Check sheet for the modelled part. Datum: model origin and axes. Units: mm. A direction names the side the tool comes from. Round coordinates to 2 decimals unless told otherwise and drop trailing zeros. Write each loop counter-clockwise with the first axis right and the second up, starting at its lowest first coordinate (ties: lowest second). Pieces come first, ordered by that corner, then holes. Notation, with made-up numbers: (10, 47) -> (16, 47) arc R18 ccw to (16, 58) -> close; hole circle Ø5 at (50.25, 10). An arc over 180 degrees is marked (long way). Write item = value, one per line.
Autodesk Inventor part; units mm, degrees
ref_plane "YZ Plane" through (0, 0, 0) normal (1, 0, 0) x (0, 1, 0)
ref_plane "XZ Plane" through (0, 0, 0) normal (0, 1, 0) x (-1, 0, 0)
ref_plane "XY Plane" through (0, 0, 0) normal (0, 0, 1) x (1, 0, 0)
sketch "Sketch1" plane through (0, 0, 0) normal (0, 1, 0) x (-1, 0, 0)
  line L0 (73.3629, -5.9836) -> (60.8629, -5.9836)
  line L1 (60.8629, -5.9836) -> (60.8629, -18.4836)
  line L2 (60.8629, -18.4836) -> (73.3629, -18.4836)
  line L3 (73.3629, -18.4836) -> (73.3629, -5.9836)
  line L4 (107.9129, -0.7336) -> (40.3129, -0.7336)
  line L5 (40.3129, -23.7336) -> (107.9129, -23.7336)
  line L6 (77.3838, -12.2336) -> (49.3838, -12.2336) construction
  line L7 (67.1129, -2.25) -> (67.1129, -23.25) construction
  line L8 (81.1129, -9.7336) -> (107.9129, -9.7336)
  line L9 (107.9129, -14.7336) -> (81.1129, -14.7336)
  line L10 (48.1129, -23.7336) -> (48.1129, -0.7336)
  line L11 (46.3129, -0.7336) -> (46.3129, -23.7336)
  line L12 (52.6129, -10.7336) -> (40.3129, -10.7336)
  line L13 (52.6129, -13.7336) -> (40.3129, -13.7336)
  line L14 (101.1129, -15.2836) -> (99.6129, -15.2836)
  line L15 (99.6129, -15.2836) -> (99.6129, -9.1836)
  line L16 (99.6129, -9.1836) -> (101.1129, -9.1836)
  line L17 (79.1129, -0.7336) -> (79.1129, -23.7336)
  line L18 (81.1129, -23.7336) -> (81.1129, -0.7336)
  line L19 (55.1129, -0.7336) -> (55.1129, -23.7336)
  line L20 (79.1129, -13.7336) -> (73.3629, -13.7336)
  line L21 (73.3629, -10.7336) -> (79.1129, -10.7336)
  line L22 (60.8629, -13.7336) -> (55.1129, -13.7336)
  line L23 (55.1129, -10.7336) -> (60.8629, -10.7336)
  line L24 (73.3629, -18.4836) -> (77.5629, -18.4836)
  line L25 (77.5629, -18.4836) -> (77.5629, -15.2836)
  line L26 (77.5629, -15.2836) -> (73.3629, -15.2836)
  line L27 (73.3629, -15.2836) -> (60.8629, -15.2836)
  line L28 (56.2629, -15.2836) -> (56.2629, -18.4836)
  line L29 (56.2629, -18.4836) -> (59.4629, -18.4836)
  line L30 (59.4629, -15.2836) -> (56.2629, -15.2836)
  line L31 (59.4629, -5.9836) -> (56.2629, -5.9836)
  line L32 (56.2629, -5.9836) -> (56.2629, -9.1836)
  line L33 (56.2629, -9.1836) -> (59.4629, -9.1836)
  line L34 (60.8629, -9.1836) -> (73.3629, -9.1836)
  line L35 (77.5629, -9.1836) -> (77.5629, -5.9836)
  line L36 (73.3629, -5.9836) -> (77.5629, -5.9836)
  line L37 (77.5629, -9.1836) -> (73.3629, -9.1836)
  line L38 (59.4629, -18.4836) -> (59.4629, -15.2836)
  line L39 (59.4629, -9.1836) -> (59.4629, -5.9836)
  line L40 (60.8629, -18.4836) -> (59.4629, -18.4836)
  line L41 (60.8629, -15.2836) -> (59.4629, -15.2836)
  line L42 (60.8629, -9.1836) -> (59.4629, -9.1836)
  line L43 (60.8629, -5.9836) -> (59.4629, -5.9836)
  line L44 (40.3129, -23.7336) -> (40.3129, -0.7336)
  line L45 (107.9129, -23.7336) -> (107.9129, -0.7336)
  line L46 (53.1129, -14.7336) -> (52.6129, -14.7336)
  line L47 (52.6129, -14.7336) -> (52.6129, -9.7336)
  line L48 (52.6129, -9.7336) -> (53.1129, -9.7336)
  line L49 (53.1129, -23.7336) -> (53.1129, -14.7336)
  line L50 (53.1129, -9.7336) -> (53.1129, -0.7336)
  line L51 (101.1129, -16.2336) -> (98.1129, -16.2336)
  line L52 (98.1129, -16.2336) -> (98.1129, -18.2336)
  line L53 (98.1129, -18.2336) -> (101.1129, -18.2336)
  line L54 (102.9129, -16.2336) -> (105.9129, -16.2336)
  line L55 (105.9129, -16.2336) -> (105.9129, -18.2336)
  line L56 (105.9129, -18.2336) -> (102.9129, -18.2336)
  line L57 (101.1129, -8.2336) -> (98.1129, -8.2336)
  line L58 (98.1129, -8.2336) -> (98.1129, -6.2336)
  line L59 (98.1129, -6.2336) -> (101.1129, -6.2336)
  line L60 (102.9129, -8.2336) -> (105.9129, -8.2336)
  line L61 (105.9129, -8.2336) -> (105.9129, -6.2336)
  line L62 (105.9129, -6.2336) -> (102.9129, -6.2336)
  line L63 (106.4404, -17.2336) -> (97.7013, -17.2336) construction
  line L64 (106, -7.2336) -> (98, -7.2336) construction
  line L65 (102.9129, -23.7336) -> (102.9129, -18.2336)
  line L66 (101.1129, -18.2336) -> (101.1129, -23.7336)
  line L67 (102.9129, -16.2336) -> (102.9129, -8.2336)
  line L68 (102.9129, -6.2336) -> (102.9129, -0.7336)
  line L69 (101.1129, -0.7336) -> (101.1129, -6.2336)
  line L70 (101.1129, -8.2336) -> (101.1129, -16.2336)
  point P0 (102.9129, -9.7336)
  point P1 (101.1129, -9.7336)
  point P2 (102.9129, -14.7336)
  point P3 (101.1129, -14.7336)
  point P4 (48.1129, -10.7336)
  point P5 (46.3129, -10.7336)
  point P6 (48.1129, -13.7336)
  point P7 (46.3129, -13.7336)
  point P8 (67.1129, -12.2336)
  point P9 (99.6129, -9.7336)
  point P10 (99.6129, -14.7336)
  dimension "d0" = 12.5
  dimension "d1" = 12.5
  dimension "d12" = 5
  dimension "d18" = 1.8
  dimension "d39" = 1.5
  dimension "d43" = 2
  dimension "d52" = 12
  dimension "d57" = 12
  dimension "d62" = 3
  dimension "d63" = 3
  dimension "d71" = 7
  dimension "d76" = 4.2
  dimension "d77" = 3.2
  dimension "d78" = 3.2
  dimension "d79" = 1.4
  dimension "d80" = 3.2
  dimension "d91" = 6
  dimension "d92" = 3
  dimension "d95" = 23
  dimension "d98" = 5
  dimension "d99" = 0.5
  dimension "d100" = 2
  dimension "d101" = 2
  dimension "d102" = 3
  dimension "d103" = 10
  dimension "d104" = 1.8
  dimension "d105" = 20
  dimension "d107" = 6.1
  dimension "d108" = 5
  dimension "d109" = 67.6
extrude "Extrusion11" add sketch "Sketch1" against normal blind 3 contours L3 L34 L1 L0 | L1 L42 L39 L43 | L3 L2 L1 L27 | L1 L40 L38 L41
extrude "Extrusion10" add sketch "Sketch1" against normal blind 6 separate body contours L0 L43 L31 L32 L33 L42 L1 L23 L19 L4 L17 L21 L3 L37 L35 L36 | L3 L27 L1 L34 | L21 L17 L20 L3 | L1 L22 L19 L23 | L20 L17 L5 L19 L22 L1 L41 L30 L28 L29 L40 L2 L24 L25 L26 L3 | L17 L4 L18 L5 | L19 L5 L49 L46 L47 L48 L50 L4 | L4 L69 L59 L58 L57 L70 L16 L15 L8 L18 | L50 L48 L47 L12 L10 L4 | L18 L9 L15 L14 L70 L51 L52 L53 L66 L5 | L4 L68 L62 L61 L60 L67 L8 L70 L57 L58 L59 L69 | L8 L15 L9 L18 | L5 L10 L13 L47 L46 L49 | L10 L12 L11 L4 | L66 L53 L52 L51 L70 L9 L67 L54 L55 L56 L65 L5 | L4 L45 L8 L67 L60 L61 L62 L68 | L15 L16 L70 L8 | L8 L70 L9 L15 | L5 L11 L13 L10 | L11 L12 L44 L4 | L12 L47 L13 L10 | L10 L13 L11 L12 | L65 L56 L55 L54 L67 L9 L45 L5 | L9 L70 L14 L15 | L8 L67 L9 L70 | L5 L44 L13 L11 | L11 L13 L44 L12 | L45 L9 L67 L8
extrude "Extrusion15" add sketch "Sketch1" along normal blind 5 contours L0 L43 L31 L32 L33 L42 L1 L23 L19 L4 L17 L21 L3 L37 L35 L36 | L21 L17 L20 L3 | L1 L22 L19 L23 | L20 L17 L5 L19 L22 L1 L41 L30 L28 L29 L40 L2 L24 L25 L26 L3 | L4 L69 L59 L58 L57 L70 L16 L15 L8 L18 | L50 L48 L47 L12 L10 L4 | L18 L9 L15 L14 L70 L51 L52 L53 L66 L5 | L8 L15 L9 L18 | L5 L10 L13 L47 L46 L49 | L4 L45 L8 L67 L60 L61 L62 L68 | L15 L16 L70 L8 | L8 L70 L9 L15 | L11 L12 L44 L4 | L12 L47 L13 L10 | L65 L56 L55 L54 L67 L9 L45 L5 | L9 L70 L14 L15 | L5 L44 L13 L11 | L11 L13 L44 L12 | L45 L9 L67 L8
extrude "Extrusion14" add sketch "Sketch1" along normal blind 3.5 contours L3 L34 L1 L0 | L3 L27 L1 L34 | L3 L2 L1 L27
extrude "Extrusion16" add sketch "Sketch1" along normal blind 20 contours L0 L43 L31 L32 L33 L42 L1 L23 L19 L4 L17 L21 L3 L37 L35 L36 | L1 L42 L39 L43 | L20 L17 L5 L19 L22 L1 L41 L30 L28 L29 L40 L2 L24 L25 L26 L3 | L1 L40 L38 L41 | L4 L69 L59 L58 L57 L70 L16 L15 L8 L18 | L50 L48 L47 L12 L10 L4 | L18 L9 L15 L14 L70 L51 L52 L53 L66 L5 | L5 L10 L13 L47 L46 L49 | L4 L45 L8 L67 L60 L61 L62 L68 | L11 L12 L44 L4 | L65 L56 L55 L54 L67 L9 L45 L5 | L5 L44 L13 L11
properties part number "Spirulina_prototype"
(1) Sectioned sample at B-B on x = -76. Enter the section's corners in (y, z), then the cut area to 3 significant figures.
Worked answers:
outline = (-6, -23.73) -> (20, -23.73) -> (20, -18.48) -> (-6, -18.48) -> close; (-6, -15.28) -> (20, -15.28) -> (20, -13.73) -> (5, -13.73) -> (5, -10.73) -> (20, -10.73) -> (20, -9.18) -> (-6, -9.18) -> close; (-6, -5.98) -> (20, -5.98) -> (20, -0.73) -> (-6, -0.73) -> close
area = 387 mm²
(2) Sectioned sample at A-A on z = -7.5. Count the separate pieces of the cut face and the enclosed holes in it, then the cut area to 3 significant figures.
Worked answers:
separate_pieces = 3
enclosed_holes = 0
area = 1,050 mm²
(3) Release check for a two-part mould opening along Z. For faces 5 (the flat face through (-100, 12, -15.284)), 6 (the flat face through (-90, 12, -14.734)), 7 (the flat face through (-46.313, 10, -15)), 8 (the flat face through (-74, 7, -23.734)) record: pulls with the +Z half, pulls with the -Z half, needs draft (parallel to the pull), parting line crosses it, or undercut.
Worked answers:
face_5 = undercut
face_6 = undercut
face_7 = needs draft
face_8 = pulls with the -Z half
(4) Material ranges on L1, parallel to Z at x = -104, y = 8.75; L2, parallel to X at y = 3, z = -1.75; L3, parallel to X at y = 7, z = -14.5, recorded low to high. Write a range as [from, to].
Worked answers:
L1 = [-23.73, -18.23], [-16.23, -14.73], [-9.73, -8.23], [-6.23, -0.73]
L2 = [-107.91, -102.91], [-101.11, -81.11], [-79.11, -55.11], [-53.11, -48.11], [-46.31, -40.31]
L3 = [-79.11, -73.36], [-60.86, -55.11], [-52.61, -48.11], [-46.31, -40.31]
(5) Sectioned sample at D-D on x = -100.5. Enter the section's corners in (y, z).
Worked answers:
outline = (-6, -23.73) -> (20, -23.73) -> (20, -18.23) -> (0, -18.23) -> (0, -16.23) -> (20, -16.23) -> (20, -15.28) -> (5, -15.28) -> (5, -9.18) -> (20, -9.18) -> (20, -8.23) -> (0, -8.23) -> (0, -6.23) -> (20, -6.23) -> (20, -0.73) -> (-6, -0.73) -> close
(6) Go/stop test with flat-tipped pins: P1, Ø1.8, axis at x = -93, z = -13.5, coming from the +Y side; P2, Ø1, axis at x = -80, y = 9, coming from the -Z side. Record where each tip stops, or that it passes through.
Worked answers:
P1 = 5
P2 = through
(7) Access from +Z, -Z, +X, -X, +Y, -Y to the whole of each face (thin tool, end or side, straight path). Record for faces 1 (the flat face through (-79.113, 10, -15)), 2 (the flat face through (-105, 5, -12)), 3 (the flat face through (-76, 12, -13.734)), 4 (the flat face through (-104, 10, -6.234)).
Worked answers:
face_1 = +Z, -Z, +Y
face_2 = -X, +Y
face_3 = +X, -X, +Y
face_4 = +Y
